Design review of the part built by this model. Coordinates are the model's own, in mm. A direction names the side the tool comes from. Coordinates: 2 decimals unless noted, no trailing zeros. Write each loop counter-clockwise with the first axis right and the second up, starting at its lowest first coordinate (ties: lowest second). Pieces come first, ordered by that corner, then holes. Notation, with made-up numbers: (20, 38) - (70, 38) arc R16 cw to (70, 53) - close; hole circle Ø2 at (87.25, -22). An arc over 180 degrees is marked (long way). Use a Markdown table: item, result.
from build123d import *

# Parameters (mm, degrees)
BOSS_EXTRUDE1_DEPTH  = 50
SKETCH2_R            = 5
BOSS_EXTRUDE2_DEPTH  = 9.5
SKETCH3_R            = 2.5
CUT_EXTRUDE1_DEPTH   = 4
FILLET1_R            = 0.5
FILLET1_OF_MIRROR2_R = 0.5


with BuildPart() as part:
    # Sketch1 → Boss-Extrude1 (new body)
    with BuildSketch(Plane(origin=(0, 0, 0), x_dir=(0, 0, -1), z_dir=(1, 0, 0))):
        Polygon((0, 0), (0, 43.5), (66.6, 43.5), (66.6, 46.5), (-3, 46.5), (-3, -3), (10, -3), (10, 0), align=None)
    extrude(amount=BOSS_EXTRUDE1_DEPTH)

    # Sketch2 → Boss-Extrude2 (add)
    with BuildSketch(Plane(origin=(50, 0, 0), x_dir=(0, 0, -1), z_dir=(1, 0, 0))):
        with Locations((71.272526987, 44.565123004)):
            Circle(SKETCH2_R)
    boss_extrude2 = extrude(amount=-BOSS_EXTRUDE2_DEPTH)

    # Sketch3 → Cut-Extrude1 (cut)
    with BuildSketch(Plane.ZY.offset(-40.5)):
        with Locations((-71.272526987, 44.565123004)):
            Circle(SKETCH3_R)
    cut_extrude1 = extrude(amount=-CUT_EXTRUDE1_DEPTH, mode=Mode.SUBTRACT)

    # Fillet1
    fillet1_edges = [part.edges().sort_by_distance(p)[0] for p in [
        (40.5, 44.565123004, -73.772526987),
    ]]
    fillet(fillet1_edges, radius=FILLET1_R)

    # Mirror2: Boss-Extrude2, Cut-Extrude1 across plane
    add(boss_extrude2.mirror(Plane(origin=(25, 0, 0), x_dir=(0, 0, 1), z_dir=(1, 0, 0))))
    add(cut_extrude1.mirror(Plane(origin=(25, 0, 0), x_dir=(0, 0, 1), z_dir=(1, 0, 0))), mode=Mode.SUBTRACT)

    # Fillet1 of Mirror2
    fillet1_of_mirror2_edges = [part.edges().sort_by_distance(p)[0] for p in [
        (9.5, 44.565123004, -73.772526987),
    ]]
    fillet(fillet1_of_mirror2_edges, radius=FILLET1_OF_MIRROR2_R)


solid = part.part
(1) Machinability: for faces 4 (the cylindrical face through (42.73, 45.32, -68.89)), 5 (the flat face through (25, -2, -10)), 6 (the flat face through (25, 0, -5)), which of the approach directions +Z, -Z, +X, -X, +Y, -Y give a long, thin tool a straight path to every point of the face, cutting with its end or side? Answer none if there is none.
Determined:
| item | result |
|---|---|
| face 4 | none |
| face 5 | -Z, +X, -X, -Y |
| face 6 | -Z, +X, -X |
(2) Take a section at C-C on z = -60.5. Write out the cut boundary in (x, y).
Determined:
| item | result |
|---|---|
| outline | (0, 43.5) - (50, 43.5) - (50, 46.5) - (0, 46.5) - close |
(3) Take a section at B-B on y = 24.5. Write out the cut boundary in (x, z).
Determined:
| item | result |
|---|---|
| outline | (0, 0) - (50, 0) - (50, 3) - (0, 3) - close |
(4) For L1, parallel to Y at x = 12.5, z = -2.5; L2, parallel to Z at x = 47.5, y = 15; L3, parallel to Y at x = 20, z = -27, list the stretches that pass through material, from the lowest coordinate up. Write a range as from..to.
Determined:
| item | result |
|---|---|
| L1 | -3..0, 43.5..46.5 |
| L2 | 0..3 |
| L3 | 43.5..46.5 |
(5) For pin 1 (3 mm diameter, centred on x = 44.5, z = -68, fed in from -Y); pin 2 (3.5 mm diameter, centred on x = 22, y = -2, fed in from -Z); pin 3 (15 mm diameter, centred on x = 17, z = -42, fed in from -Y), all flat-tipped, find the tip position at first contact; note any pin that passes through.
Determined:
| item | result |
|---|---|
| pin 1 | y = 39.89 |
| pin 2 | z = -10 |
| pin 3 | y = 43.5 |
(6) Take a section at A-A on x = 43. Write out the cut boundary in (y, z), and give its area (3 significant figures).
Determined:
| item | result |
|---|---|
| outline | (-3, -10) - (0, -10) - (0, 0) - (43.5, 0) - (43.5, -66.39) arc R5 ccw (long way) to (46.34, -66.6) - (46.5, -66.6) - (46.5, 3) - (-3, 3) - close; hole circle Ø5 at (44.57, -71.27) |
| area | 437 mm2 |
(7) Draft analysis for pull direction Y (two halves, no side actions). For faces 1 (the flat face through (25, 22, 3)), 2 (the flat face through (25, 46.5, -32)), 3 (the flat face through (44.5, 45, -71)), state which applies: +Y half, -Y half, draft (parallel to the pull), parting line (faces both ways), or undercut.
Determined:
| item | result |
|---|---|
| face 1 | draft |
| face 2 | +Y half |
| face 3 | undercut |
